The listing builds one solid part. Answer for the finished solid, in the listing's coordinates (mm). Round coordinates to 2 decimals unless told otherwise and drop trailing zeros. Loops run counter-clockwise (first coordinate to the right, second up) from the corner with the lowest first, then second, coordinate; pieces in that order, holes last. Notation, with made-up numbers: M 54,66.25 L 70,66.25 A20 cw 70,86.25 Z; hole C -8.75,58 d5. An arc over 180 degrees is marked long. Answer as a JSON object with one key per item and string values.
```python
from build123d import *

# Parameters (mm, degrees)
BOX_W        = 15
BOX_H        = 5
BOX_DEPTH    = 15
SKETCH_R     = 2.1
POCKET_DEPTH = 5


with BuildPart() as part:
    # Box → Box (new body)
    with BuildSketch(Plane.XY):
        with Locations((7.5, 2.5)):
            Rectangle(BOX_W, BOX_H)
    extrude(amount=BOX_DEPTH)

    # Sketch → Pocket (cut)
    with BuildSketch(Plane.XZ):
        with Locations((7.5, 7.5)):
            Circle(SKETCH_R)
    extrude(amount=-POCKET_DEPTH, mode=Mode.SUBTRACT)


solid = part.part
```
Item 1: The part is cut by section B-B (x = 7.5). Give the vertices of the cut face in (y, z).
Values follow:
{"outline": "M 0,0 L 5,0 L 5,5.4 L 0,5.4 Z; M 0,9.6 L 5,9.6 L 5,15 L 0,15 Z"}
Item 2: Straight lines are drawn through the part: line 1 (Z direction, x = 7.5, y = 3.5); line 2 (Z direction, x = 6.25, y = 1.95); line 3 (X direction, y = 1.8, z = 9). For each, find the intervals that lie inside material, in ascending order.
Values follow:
{"line 1": "0 to 5.4, 9.6 to 15", "line 2": "0 to 5.81, 9.19 to 15", "line 3": "0 to 6.03, 8.97 to 15"}
Item 3: The part is cut by section C-C (y = 2.75). Give the vertices of the cut face in (x, z), then the cut area to 3 significant figures.
Values follow:
{"outline": "M 0,0 L 15,0 L 15,15 L 0,15 Z; hole C 7.5,7.5 d4.2", "area": "211 mm^2"}
Item 4: The part is cut by section A-A (z = 7.5). Give the vertices of the cut face in (x, y), then the cut area to 3 significant figures.
Values follow:
{"outline": "M 0,0 L 5.4,0 L 5.4,5 L 0,5 Z; M 9.6,0 L 15,0 L 15,5 L 9.6,5 Z", "area": "54.0 mm^2"}
Item 5: Determine the mould class of faces 1 (the face through (7.227, 2.465, 9.582)), 2 (the face through (7, 3, 0)), 3 (the face through (15, 2, 7)) for opening direction Z: released by +Z, released by -Z, zero draft, split by the parting line, or undercut.
Values follow:
{"face 1": "undercut", "face 2": "released by -Z", "face 3": "zero draft"}
